Verification items for the finished model (mm, model axes). A direction names the side the tool comes from. Coordinates: 2 decimals unless noted, no trailing zeros. Order: outer loops, then holes, each group sorted by start corner. A loop starts at its lowest first (then second) coordinate and runs counter-clockwise, first axis right, second up. Notation, with made-up numbers: (-5.75, -16) -> (21.25, -16) arc R23 cw to (21.25, -6) -> close; hole circle Ø4 at (-8, 48.25). An arc over 180 degrees is marked (long way). Write each question's results on one line, items separated by ' | '. Start each with the question number.
(1) Cross-section at A-A on x = 14.5. Enter the section's corners in (y, z).
(2) Cross-section at D-D on x = 35. Enter the section's corners in (y, z), and give its area (3 significant figures).
(3) Draft check along X on faces 6 (the flat face through (0, 0, 12)), 7 (the flat face through (-2, -94, 12)), 8 (the flat face through (-50, -94, 12)), 9 (the flat face through (50, -94, 12)). Enter one of: +X half, -X half, draft (parallel to the pull), parting line (faces both ways), or undercut.
(4) Cross-section at B-B on z = 10.25. Enter the section's corners in (x, y).
(5) Set-up check for faces 1 (the flat face through (0, -190, 12)), 2 (the flat face through (-1, -94, 0)), 3 (the cylindrical face through (-36.75, -162.74, 24.01)), 4 (the cylindrical face through (31.269, -7.547, 0.986)), 5 (the flat face through (2, -94, 12)): record each of +Z, -Z, +X, -X, +Y, -Y from which the full face is reachable in a straight line by a thin tool's end or side.
(6) Cross-section at C-C on y = -56. Enter the section's corners in (x, z), and give its area (3 significant figures).
(7) Go/stop test with flat-tipped pins: pin 1 (3.5 mm diameter, centred on x = 30, y = -9.99, fed in from -Z); pin 2 (4 mm diameter, centred on x = 35, y = -160, fed in from +Z). Record where each tip stops, or that it passes through.
(8) Thickness scan on probe 1 along Y at (x, z) = (-30, 1.3); probe 2 along X at (y, z) = (-81, 16.5); probe 3 along X at (y, z) = (-160, 23.7). Record the ranges inside material, lowest first. Write a range as [from, to].
```python
from build123d import *

# Parameters (mm, degrees)
SKETCH_W        = 100
SKETCH_H        = 25
SKETCH_W_2      = 46
SKETCH_H_2      = 21
PAD_DEPTH       = 190
SKETCH001_R     = 2.75
POCKET_DEPTH    = 2
SKETCH002_R     = 3.25
POCKET001_DEPTH = 2


with BuildPart() as part:
    # Sketch → Pad (new body)
    with BuildSketch(Plane.XZ):
        with Locations((0, 12.5)):
            Rectangle(SKETCH_W, SKETCH_H)
        with Locations((-25, 12.5)):
            Rectangle(SKETCH_W_2, SKETCH_H_2, mode=Mode.SUBTRACT)
        with Locations((25, 12.5)):
            Rectangle(SKETCH_W_2, SKETCH_H_2, mode=Mode.SUBTRACT)
    extrude(amount=PAD_DEPTH)

    # Sketch001 (on Face3 of Pad) → Pocket (cut)
    with BuildSketch(Plane(origin=(0, 0, 0), x_dir=(1, 0, 0), z_dir=(0, 0, -1))):
        with Locations((-29.982102, 89.999998)):
            Circle(SKETCH001_R)
        with Locations((30.017897, 89.986574)):
            Circle(SKETCH001_R)
        with Locations((-30, 10)):
            Circle(SKETCH001_R)
        with Locations((29.999998, 9.986576)):
            Circle(SKETCH001_R)
    extrude(amount=-POCKET_DEPTH, mode=Mode.SUBTRACT)

    # Sketch002 (on Face1 of Pocket) → Pocket001 (cut)
    with BuildSketch(Plane(origin=(0, 0, 25), x_dir=(-1, 0, 0), z_dir=(0, 0, 1))):
        with Locations((-35, 180)):
            Circle(SKETCH002_R)
        with Locations((35, 180)):
            Circle(SKETCH002_R)
        with Locations((-35, 160)):
            Circle(SKETCH002_R)
        with Locations((35, 160)):
            Circle(SKETCH002_R)
    extrude(amount=-POCKET001_DEPTH, mode=Mode.SUBTRACT)


solid = part.part
```
Results are:
1) outline: (-190, 0) -> (0, 0) -> (0, 2) -> (-190, 2) -> close; (-190, 23) -> (0, 23) -> (0, 25) -> (-190, 25) -> close
2) outline: (-190, 0) -> (0, 0) -> (0, 2) -> (-190, 2) -> close; (-190, 23) -> (-183.25, 23) -> (-183.25, 25) -> (-190, 25) -> close; (-176.75, 23) -> (-163.25, 23) -> (-163.25, 25) -> (-176.75, 25) -> close; (-156.75, 23) -> (0, 23) -> (0, 25) -> (-156.75, 25) -> close | area: 734 mm2
3) face 6: draft | face 7: undercut | face 8: -X half | face 9: +X half
4) outline: (-50, -190) -> (-48, -190) -> (-48, 0) -> (-50, 0) -> close; (-2, -190) -> (2, -190) -> (2, 0) -> (-2, 0) -> close; (48, -190) -> (50, -190) -> (50, 0) -> (48, 0) -> close
5) face 1: +Z, -Z, +X, -X, -Y | face 2: -Z, +X, -X, +Y, -Y | face 3: +Z | face 4: -Z | face 5: +Y, -Y
6) outline: (-50, 0) -> (50, 0) -> (50, 25) -> (-50, 25) -> close; hole (-48, 2) -> (-2, 2) -> (-2, 23) -> (-48, 23) -> close; hole (2, 2) -> (48, 2) -> (48, 23) -> (2, 23) -> close | area: 568 mm2
7) pin 1: stops at z = 23 | pin 2: stops at z = 2
8) probe 1: y = [-190, -92.75], [-87.25, -12.75], [-7.25, 0] | probe 2: x = [-50, -48], [-2, 2], [48, 50] | probe 3: x = [-50, -38.25], [-31.75, 31.75], [38.25, 50]
